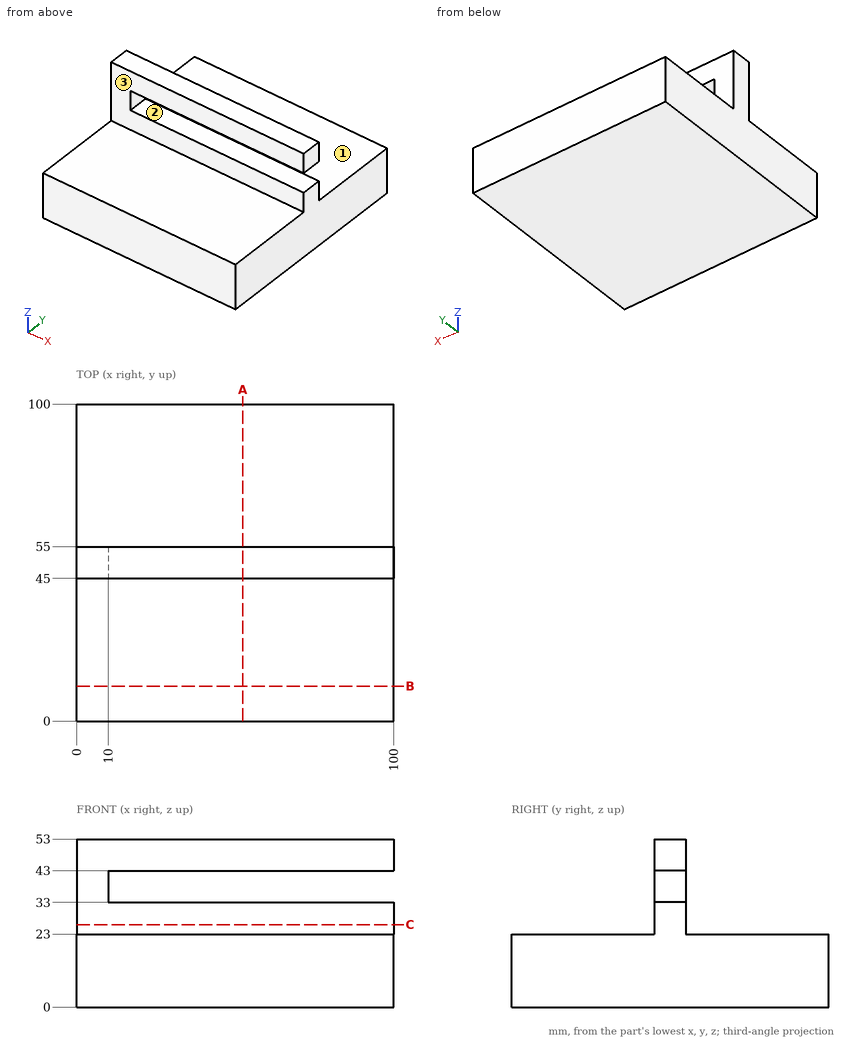
Here's the drawing with two shaded views (mm, measured from the low corner). I have some questions. A direction names the side the tool comes from. Coordinates: 2 decimals unless noted, no trailing zeros. Write each loop counter-clockwise with the first axis right and the second up, starting at its lowest first coordinate (ties: lowest second). Pieces come first, ordered by that corner, then holes.
Item 1: I want a section at A-A on x = 52.5. Write out the boundary of the cut face in (y, z).
Item 2: I want a section at C-C on z = 26. Write out the boundary of the cut face in (x, y), and give its area (3 significant figures).
Item 3: If I drill on line 1 (Z direction, x = 25, y = 91.5); line 2 (Y direction, x = 8.5, z = 39.5), over which ranges is the centre line in solid material (lowest first)?
Item 4: I want a section at B-B on y = 11. Write out the boundary of the cut face in (x, z).
Item 5: Will these pins go through, and if not, where does the flat tip stop? pin 1 (8 mm diameter, centred on x = 55.5, z = 33, fed in from -Y); pin 2 (15 mm diameter, centred on x = 51.5, z = 34.5, fed in from +Y); pin 3 (2 mm diameter, centred on x = 14.5, y = 76.5, fed in from +Z).
Item 6: On a 3-axis mill with a long thin cutter (end or side, diameter ignored), from which of +Z, -Z, +X, -X, +Y, -Y can I reach the whole of each face in a straight line? I mean the marked faces 1, 2 and 3. Say none if no direction works.
Findings below:
1. outline: (0, 0) - (100, 0) - (100, 23) - (55, 23) - (55, 33) - (45, 33) - (45, 23) - (0, 23) - close; (45, 43) - (55, 43) - (55, 53) - (45, 53) - close
2. outline: (0, 45) - (100, 45) - (100, 55) - (0, 55) - close
2. area: 1,000 mm2
3. line 1: z = 0 to 23
3. line 2: y = 45 to 55
4. outline: (0, 0) - (100, 0) - (100, 23) - (0, 23) - close
5. pin 1: stops at y = 45
5. pin 2: stops at y = 55
5. pin 3: stops at z = 23
6. face 1: +Z, +X, -X, +Y
6. face 2: +X, +Y, -Y
6. face 3: +Z, +X, -X, -Y
